Work out the finished part from the listing and answer in its coordinate system (mm). Face numbers are marked on the shaded views. Give positions to 0.01 mm unless a question says otherwise; leave off trailing zeros. Order: outer loops, then holes, each group sorted by start corner. A loop starts at its lowest first (then second) coordinate and runs counter-clockwise, first axis right, second up.
```python
from build123d import *

# Parameters (mm, degrees)
ESQUISSE1_R                         = 56.125
ESQUISSE1_R_2                       = 41.125
BOSS_EXTRU_1_DEPTH                  = 19.75
BOSS_EXTRU_2_REACH                  = 83.793
BOSS_EXTRU_2_END_RADIUS             = 41.125
ESQUISSE2_W                         = 6.583333334
ESQUISSE2_H                         = 6.583333334
BOSS_EXTRU_2_DIRECTION_2_REACH      = 83.793
BOSS_EXTRU_2_DIRECTION_2_END_RADIUS = 41.125
R_P_TITION_CIRCULAIRE1_COUNT        = 2
R_P_TITION_CIRCULAIRE1_ANGLE        = 90
ESQUISSE5_W                         = 6.583333334
ESQUISSE5_H                         = 6.583333334
BOSS_EXTRU_3_DEPTH                  = 30
ESQUISSE6_W                         = 6.583333334
ESQUISSE6_H                         = 6.583333334
BOSS_EXTRU_4_DEPTH                  = 100


with BuildPart() as part:
    # Esquisse1 → Boss.-Extru.1 (new body)
    with BuildSketch(Plane.XY):
        Circle(ESQUISSE1_R)
        Circle(ESQUISSE1_R_2, mode=Mode.SUBTRACT)
    extrude(amount=BOSS_EXTRU_1_DEPTH)

    # Boss.-Extru.2: up to this cylinder (the profile starts inside it)
    boss_extru_2_end = Plane(origin=(0, 0, 9.875), z_dir=(0, 0, -1)) * Cylinder(BOSS_EXTRU_2_END_RADIUS, 250.836, mode=Mode.PRIVATE)
    # Esquisse2 → Boss.-Extru.2 (add, up to the surface)
    with BuildSketch(Plane(origin=(0, 0, 0), x_dir=(0, 0, -1), z_dir=(1, 0, 0)), mode=Mode.PRIVATE) as boss_extru_2_sk1:
        with Locations((-9.875, 0)):
            Rectangle(ESQUISSE2_W, ESQUISSE2_H)
    boss_extru_2_tool1 = extrude(boss_extru_2_sk1.sketch, amount=BOSS_EXTRU_2_REACH, mode=Mode.PRIVATE) & boss_extru_2_end
    boss_extru_2 = boss_extru_2_tool1.solids().sort_by_distance((0, 0, 9.875))[0]
    add(boss_extru_2)

    # Boss.-Extru.2 direction 2: up to this cylinder (the profile starts inside it)
    boss_extru_2_direction_2_end = Plane(origin=(0, 0, 9.875), z_dir=(0, 0, -1)) * Cylinder(BOSS_EXTRU_2_DIRECTION_2_END_RADIUS, 250.836, mode=Mode.PRIVATE)
    # Esquisse2 → Boss.-Extru.2 direction 2 (add, up to the surface)
    with BuildSketch(Plane(origin=(0, 0, 0), x_dir=(0, 0, -1), z_dir=(1, 0, 0)), mode=Mode.PRIVATE) as boss_extru_2_direction_2_sk1:
        with Locations((-9.875, 0)):
            Rectangle(ESQUISSE2_W, ESQUISSE2_H)
    boss_extru_2_direction_2_tool1 = extrude(boss_extru_2_direction_2_sk1.sketch, amount=-BOSS_EXTRU_2_DIRECTION_2_REACH, mode=Mode.PRIVATE) & boss_extru_2_direction_2_end
    boss_extru_2_direction_2 = boss_extru_2_direction_2_tool1.solids().sort_by_distance((0, 0, 9.875))[0]
    add(boss_extru_2_direction_2)
    boss_extru_2 = boss_extru_2 + boss_extru_2_direction_2  # both directions under the feature's name, for the pattern or mirror that repeats it

    # Répétition circulaire1: Boss.-Extru.2 ×2 about axis
    r_p_tition_circulaire1_axis = Axis((0, 0, 32.118593888), (0, 0, -1))
    for i in range(1, R_P_TITION_CIRCULAIRE1_COUNT):
        add(boss_extru_2.rotate(r_p_tition_circulaire1_axis, i * R_P_TITION_CIRCULAIRE1_ANGLE / (R_P_TITION_CIRCULAIRE1_COUNT - 1)))

    # Esquisse5 → Boss.-Extru.3 (add)
    with BuildSketch(Plane(origin=(0, 0, 6.583333333), x_dir=(-1, 0, 0), z_dir=(0, 0, -1))):
        Rectangle(ESQUISSE5_W, ESQUISSE5_H)
    boss_extru_3 = extrude(amount=BOSS_EXTRU_3_DEPTH)

    # Esquisse6 → Boss.-Extru.4 (add)
    with BuildSketch(Plane.ZY.offset(3.291666667)):
        with Locations((-20.125, 0)):
            Rectangle(ESQUISSE6_W, ESQUISSE6_H)
    boss_extru_4 = extrude(amount=BOSS_EXTRU_4_DEPTH)

    # Symétrie1: Boss.-Extru.3, Boss.-Extru.4 across plane
    add(boss_extru_3.mirror(Plane(origin=(0, 0, 9.875), x_dir=(1, 0, 0), z_dir=(0, 0, -1))))
    add(boss_extru_4.mirror(Plane(origin=(0, 0, 9.875), x_dir=(1, 0, 0), z_dir=(0, 0, -1))))


solid = part.part
```
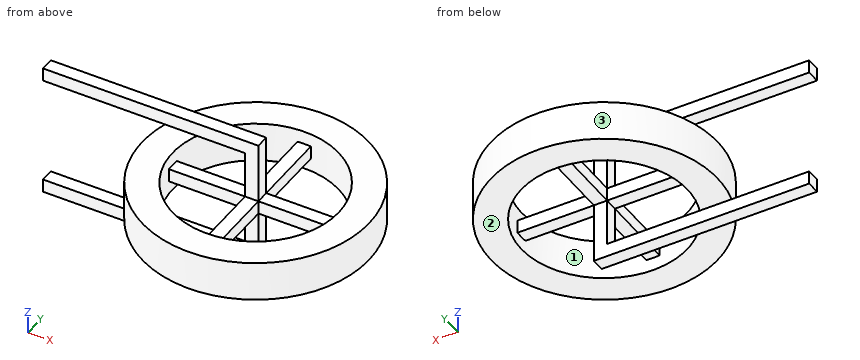
1. The part is cut by section D-D (x = -54). Write down the section's boundary in (y, z), then the cut area to 3 significant figures.
Findings below:
outline: (-15.3, 0) - (15.3, 0) - (15.3, 19.75) - (-15.3, 19.75) - close; (-3.29, -23.42) - (3.29, -23.42) - (3.29, -16.83) - (-3.29, -16.83) - close; (-3.29, 36.58) - (3.29, 36.58) - (3.29, 43.17) - (-3.29, 43.17) - close
area: 691 mm2
2. The part is cut by section A-A (x = -90). Write down the section's boundary in (y, z), then the cut area to 3 significant figures.
Findings below:
outline: (-3.29, -23.42) - (3.29, -23.42) - (3.29, -16.83) - (-3.29, -16.83) - close; (-3.29, 36.58) - (3.29, 36.58) - (3.29, 43.17) - (-3.29, 43.17) - close
area: 86.7 mm2
3. The part is cut by section B-B (y = -26). Write down the section's boundary in (x, z), then the cut area to 3 significant figures.
Findings below:
outline: (-49.74, 0) - (-31.86, 0) - (-31.86, 19.75) - (-49.74, 19.75) - close; (-3.29, 6.58) - (3.29, 6.58) - (3.29, 13.17) - (-3.29, 13.17) - close; (31.86, 0) - (49.74, 0) - (49.74, 19.75) - (31.86, 19.75) - close
area: 749 mm2
4. Given P1, Ø5.5, axis at y = 0.5, z = -9.5, coming from the -X side; P2, Ø1, axis at x = 3, y = -39.5, coming from the -Z side; P3, Ø10, axis at x = 16.5, y = -42, coming from the -Z side; P4, Ø4, axis at x = -52.5, z = -13.5, coming from the +Y side, each flat-ended and moving along its own axis, determine where each tip first touches the part or whether it passes through.
Findings below:
P1: stops at x = -3.29
P2: stops at z = 6.58
P3: stops at z = 0
P4: passes through
5. The mould has two halves that part along X. Classify the marked faces 1, 2 and 3: pulls with the +X half, pulls with the -X half, needs draft (parallel to the pull), parting line crosses it, or undercut.
Findings below:
face 1: undercut
face 2: needs draft
face 3: parting line crosses it
6. Straight lines are drawn through the part: probe 1 along Y at (x, z) = (0, 5) (3 decimals); probe 2 along Z at (x, y) = (-37, 23); probe 3 along Y at (x, z) = (-1, -18.5). For each, find the intervals that lie inside material, in ascending order.
Findings below:
probe 1: y = -56.125 to -41.125, -3.292 to 3.292, 41.125 to 56.125
probe 2: z = 0 to 19.75
probe 3: y = -3.29 to 3.29
7. The part is cut by section C-C (x = 0). Write down the section's boundary in (y, z) (3 decimals).
Findings below:
outline: (-56.125, 0) - (-41.125, 0) - (-41.125, 6.583) - (-3.292, 6.583) - (-3.292, -23.417) - (3.292, -23.417) - (3.292, 6.583) - (41.125, 6.583) - (41.125, 0) - (56.125, 0) - (56.125, 19.75) - (41.125, 19.75) - (41.125, 13.167) - (3.292, 13.167) - (3.292, 43.167) - (-3.292, 43.167) - (-3.292, 13.167) - (-41.125, 13.167) - (-41.125, 19.75) - (-56.125, 19.75) - close
